Design review of the part built by this model. Coordinates are the model's own, in mm. Round coordinates to 2 decimals unless told otherwise and drop trailing zeros. Loops run counter-clockwise (first coordinate to the right, second up) from the corner with the lowest first, then second, coordinate; pieces in that order, holes last. Notation, with made-up numbers: (-40, -8.5) -> (17, -8.5) arc R28 cw to (17, 25.5) -> close; hole circle Ø2 at (69, 50). An arc over 180 degrees is marked (long way). Answer as CSV lines item,"result". Start each with the question number.
(1) Take a section at A-A, the plane y = -3.25. Write out the cut boundary in (x, z).
(2) Take a section at B-B, the plane x = 29. Write out the cut boundary in (y, z).
(3) For P1, Ø5, axis at x = 17, y = -19.5, coming from the +Z side; P2, Ø1.5, axis at x = 41.5, y = -16, coming from the +Z side, all flat-tipped, find the tip position at first contact; note any pin that passes through.
(4) To check wall thickness, follow line 1 (X direction, y = -17.25, z = 25); line 2 (X direction, y = -19.25, z = 12.5); line 3 (Z direction, x = 42, y = -20.75). State the ranges of each line that lie inside material, in increasing order. Write a range as from..to.
(5) Take a section at D-D, the plane z = 24.5. Write out the cut boundary in (x, y), and give its area (3 significant figures).
(6) Take a section at C-C, the plane z = 12.75. Write out the cut boundary in (x, y).
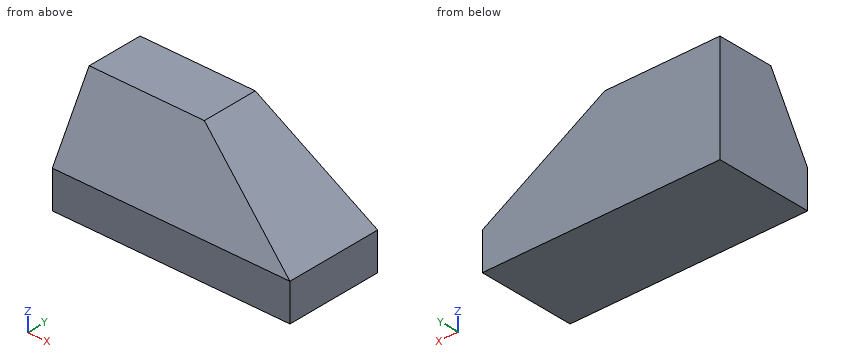
from build123d import *

# Parameters (mm, degrees)
F1_DEPTH = 27
F3_DEPTH = 66.001


with BuildPart() as f1:
    # F0 (on Front) → F1 (new body)
    with BuildSketch(Plane.XZ):
        Polygon((0, 30), (0, 0), (66, 0), (66, 10.370091), (32, 30), align=None)
    extrude(amount=F1_DEPTH)

    # F2 (on face) → F3 (cut, through all)
    with BuildSketch(Plane(origin=(0, 0, 0), x_dir=(0, -1, 0), z_dir=(-1, 0, 0))):
        Polygon((15.666667, 30), (27, 10.370091), (27, 30), align=None)
    extrude(amount=-F3_DEPTH, mode=Mode.SUBTRACT)


solid = f1.part
The answers:
1,outline,"(0, 0) -> (66, 0) -> (66, 10.37) -> (32, 30) -> (0, 30) -> close"
2,outline,"(-27, 0) -> (0, 0) -> (0, 30) -> (-15.67, 30) -> (-27, 10.37) -> close"
3,P1,"z = 27.69"
3,P2,"z = 24.95"
4,line 1,"0..40.66"
4,line 2,"0..62.31"
4,line 3,"0..21.2"
5,outline,"(0, -18.84) -> (41.53, -18.84) -> (41.53, 0) -> (0, 0) -> close"
5,area,"782 mm²"
6,outline,"(0, -25.63) -> (61.88, -25.63) -> (61.88, 0) -> (0, 0) -> close"
